Geometry check sheet. Reference: the model listing, model coordinates, mm. Face numbers are marked on the shaded views. A direction names the side the tool comes from. Coordinates: 2 decimals unless noted, no trailing zeros. Order: outer loops, then holes, each group sorted by start corner. A loop starts at its lowest first (then second) coordinate and runs counter-clockwise, first axis right, second up.
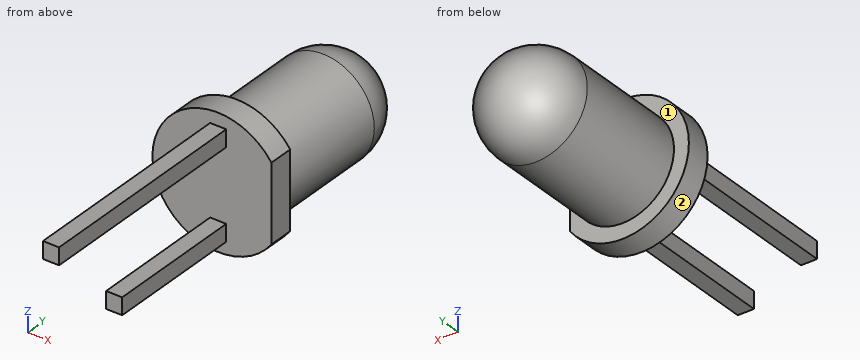
Autodesk Inventor part; units mm, degrees
ref_plane "YZ Plane" through (0, 0, 0) normal (1, 0, 0) x (0, 1, 0)
ref_plane "XZ Plane" through (0, 0, 0) normal (0, 1, 0) x (-1, 0, 0)
ref_plane "XY Plane" through (0, 0, 0) normal (0, 0, 1) x (1, 0, 0)
sketch "Sketch1" plane through (0, 0, 0) normal (0, 0, 1) x (1, 0, 0)
  line L0 (0, 0) -> (1.8733, 0)
  line L1 (1.8733, 0) -> (1.8733, 0.7112)
  line L2 (1.8733, 0.7112) -> (1.4478, 0.7112)
  line L3 (1.4478, 0.7112) -> (1.4478, 4.0005)
  arc A0 (1.4478, 4.0005) -> (0, 5.4483) centre (0, 4.0005) ccw
  line L4 (0, 5.4483) -> (0, 0)
  dimension "d0" = 1.4478
  dimension "d1" = 0.7112
  dimension "d2" = 1.8733
  dimension "d3" = 5.4483
revolve "Revolution1" add sketch "Sketch1" angle 360 about axis through (0, 5.4483, 0) along (0, -1, 0)
sketch "Sketch2" plane through (0, 0, 0) normal (0, -1, 0) x (1, 0, 0)
  line L0 (4.2518, 2.7248) -> (1.5176, 2.7248)
  line L1 (1.5176, 2.7248) -> (1.5177, -2.7614)
  line L2 (1.5177, -2.7614) -> (4.2518, -2.7614)
  line L3 (4.2518, -2.7614) -> (4.2518, 2.7248)
  circle A0 centre (0, 0) radius 1.8732
  dimension "d5" = 3.3909
extrude "Extrusion1" cut sketch "Sketch2" against normal blind 25.4 contours L3 L2 L1 A0 L0 | A0 L1 picked at (1.5825, -0.2532)
sketch "Sketch3" plane through (0, 0, 0) normal (0, -1, 0) x (1, 0, 0)
  line L0 (-0.2286, -1.0287) -> (0.2286, -1.0287)
  line L1 (0.2286, -1.0287) -> (0.2286, -1.5113)
  line L2 (0.2286, -1.5113) -> (-0.2286, -1.5113)
  line L3 (-0.2286, -1.5113) -> (-0.2286, -1.0287)
  line L4 (-0.2286, 1.5113) -> (0.2286, 1.5113)
  line L5 (0.2286, 1.5113) -> (0.2286, 1.0287)
  line L6 (0.2286, 1.0287) -> (-0.2286, 1.0287)
  line L7 (-0.2286, 1.0287) -> (-0.2286, 1.5113)
  line L8 (0, 0) -> (0, 1.0287)
  line L9 (0, 0) -> (0, -1.0287)
  dimension "d13" = 0.4572
  dimension "d14" = 0.4826
  dimension "d15" = 3.0226
extrude "Extrusion2" add sketch "Sketch3" along normal blind 6.35
sketch "Sketch5" plane through (0.2286, -6.35, -1.0287) normal (1, 0, 0) x (0, 0, -1)
  line L0 (1.6967, -0.6432) -> (-0.5604, -0.6432)
  line L1 (-0.5604, -0.6432) -> (-0.5604, 2.3982)
  line L2 (-0.5604, 2.3982) -> (1.6967, 2.3982)
  line L3 (1.6967, 2.3982) -> (1.6967, -0.6432)
  point P0 (-1.0287, 6.35)
extrude "Extrusion3" cut sketch "Sketch5" against normal blind 25.4
properties part number "LED"
Item 1: Sectioned sample at B-B (x = 0). Record the cut outline in (y, z).
Item 2: Sectioned sample at C-C (z = -0.65). Record the cut outline in (x, y), and give its area (3 significant figures).
Item 3: Sectioned sample at D-D (y = -5). Record the cut outline in (x, z), and give its area (3 significant figures).
Item 4: Sectioned sample at A-A (y = -3.5). Record the cut outline in (x, z).
Item 5: Depth check by flat-ended pin: P1, Ø1, axis at x = -0.5, y = -2.5, coming from the -Z side; P2, Ø0.5, axis at x = 0, y = -1.5, coming from the +Z side; P3, Ø1.5, axis at x = -0.5, y = 2.5, coming from the -Z side. Enter the tip coordinate at first touch or a pass-through.
Item 6: Thickness scan on line 1 along Z through (x, y) = (-0.1, -0.5); line 2 along Y through (x, z) = (-1.5, 0.5); line 3 along Y through (x, z) = (0.95, -0.4). Record the ranges inside material, lowest first.
Item 7: Tool access check on the marked faces 1 and 2. Record the directions out of +Z, -Z, +X, -X, +Y, -Y that give a thin tool (end or side, any length) a straight path to the whole face; none if there is none.
Geometry check:
1. outline: (-6.35, 1.03) - (0, 1.03) - (0, -1.03) - (-3.95, -1.03) - (-3.95, -1.51) - (0, -1.51) - (0, -1.87) - (0.71, -1.87) - (0.71, -1.45) - (4, -1.45) arc R1.45 ccw to (4, 1.45) - (0.71, 1.45) - (0.71, 1.87) - (0, 1.87) - (0, 1.51) - (-6.35, 1.51) - close
2. outline: (-1.76, 0) - (1.52, 0) - (1.52, 0.71) - (1.29, 0.71) - (1.29, 4) arc R1.29 ccw to (-1.29, 4) - (-1.29, 0.71) - (-1.76, 0.71) - close
2. area: 13.5 mm2
3. outline: (-0.23, 1.03) - (0.23, 1.03) - (0.23, 1.51) - (-0.23, 1.51) - close
3. area: 0.221 mm2
4. outline: (-0.23, -1.51) - (0.23, -1.51) - (0.23, -1.03) - (-0.23, -1.03) - close; (-0.23, 1.03) - (0.23, 1.03) - (0.23, 1.51) - (-0.23, 1.51) - close
5. P1: stops at z = -1.51
5. P2: stops at z = 1.51
5. P3: stops at z = -1.45
6. line 1: z = -1.51 to -1.03, 1.03 to 1.51
6. line 2: y = 0 to 0.71
6. line 3: y = 0 to 5.02
7. face 1: +Y
7. face 2: +Y, -Y
